Answer from the drawing. Dimensions are ordinates in mm from the lowest x, y and z of the part. A direction names the side the tool comes from. Round coordinates to 2 decimals unless told otherwise and drop trailing zeros. Write each loop counter-clockwise with the first axis right and the second up, starting at its lowest first coordinate (ties: lowest second). Pieces come first, ordered by that corner, then holes. Notation, with made-up numbers: (-39, -27.5) -> (-8, -27.5) arc R11 ccw to (-8, -12.5) -> close; hole circle Ø10 at (74.25, 73.25). An arc over 180 degrees is marked (long way). Return JSON: item names as keys, results as strings. Group by question number.
(1) Given pin 1 (1.6 mm diameter, centred on x = 4.5, z = 9.5, fed in from -Y), flat-ended and moving along its own axis, determine where the tip first touches the part or whether it passes through.
(2) A cutting plane is placed at C-C on x = 5.5. Give the vertices of the cut face in (y, z).
(3) The mould has two halves that part along X. Classify the marked faces 3, 4 and 5: released by +X, released by -X, zero draft, split by the parting line, or undercut.
(4) Straight lines are drawn through the part: line 1 (Z direction, x = 4.25, y = 0.7); line 2 (X direction, y = 1.8, z = 5); line 3 (Y direction, x = 3.75, z = 9.5). For each, find the intervals that lie inside material, in ascending order.
(5) A cutting plane is placed at B-B on y = 1.7. Give the vertices of the cut face in (x, z).
(6) A cutting plane is placed at A-A on z = 10.5. Give the vertices of the cut face in (x, y).
(7) For the marked faces 1 and 2, determine the directions among +Z, -Z, +X, -X, +Y, -Y from which every point of the face is accessible in a straight line to the end or side of a thin tool.
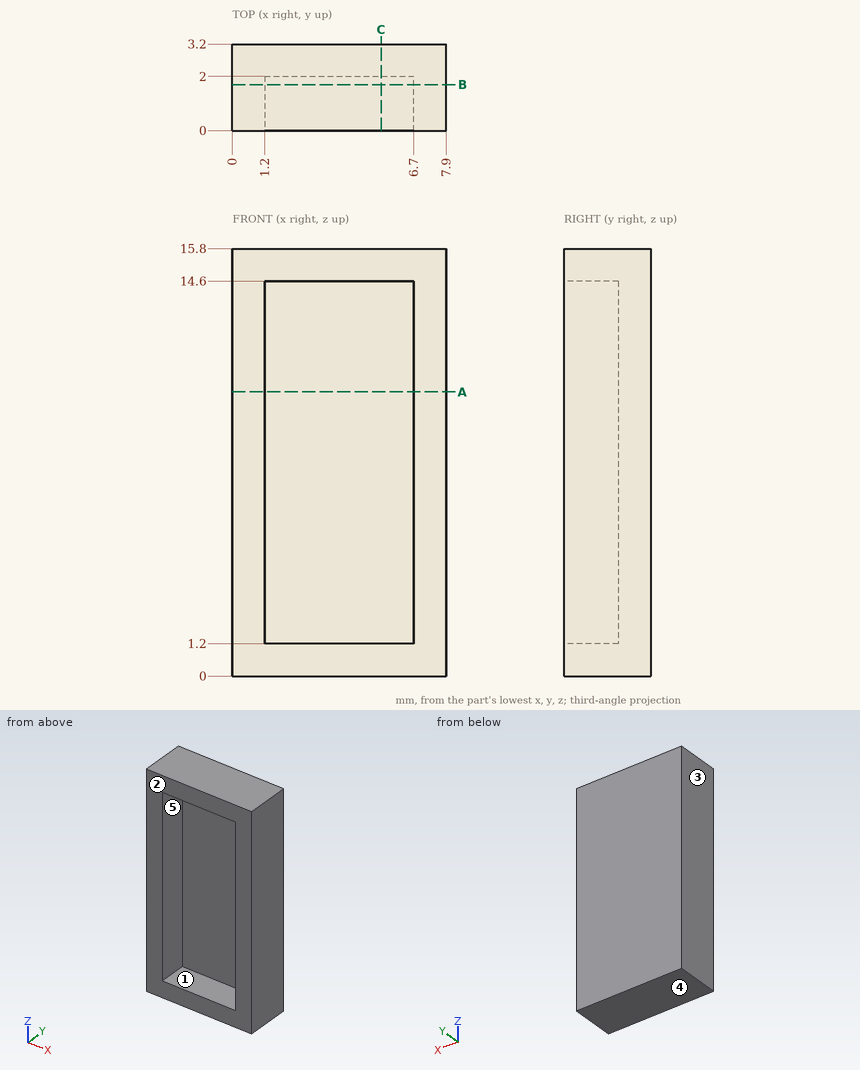
Checks:
{
 "1": {"pin 1": "stops at y = 2"},
 "2": {"outline": "(0, 0) -> (3.2, 0) -> (3.2, 15.8) -> (0, 15.8) -> (0, 14.6) -> (2, 14.6) -> (2, 1.2) -> (0, 1.2) -> close"},
 "3": {"face 3": "released by -X", "face 4": "zero draft", "face 5": "undercut"},
 "4": {"line 1": "z = 0 to 1.2, 14.6 to 15.8", "line 2": "x = 0 to 1.2, 6.7 to 7.9", "line 3": "y = 2 to 3.2"},
 "5": {"outline": "(0, 0) -> (7.9, 0) -> (7.9, 15.8) -> (0, 15.8) -> close; hole (1.2, 1.2) -> (6.7, 1.2) -> (6.7, 14.6) -> (1.2, 14.6) -> close"},
 "6": {"outline": "(0, 0) -> (1.2, 0) -> (1.2, 2) -> (6.7, 2) -> (6.7, 0) -> (7.9, 0) -> (7.9, 3.2) -> (0, 3.2) -> close"},
 "7": {"face 1": "-Y", "face 2": "+Z, -Z, +X, -X, -Y"}
}
